Autodesk Fusion 360 part; units mm, degrees
sketch "Sketch1" plane through (0, 0, 0) normal (1, 0, 0) x (0, 1, 0)
  line L0 (28, -18) -> (-28, -18)
  line L1 (-28, 18) -> (28, 18)
  line L2 (28, -18) -> (-28, 18) construction
  line L3 (-28, -18) -> (28, 18) construction
  circle A0 centre (-28, 0) radius 8
  circle A1 centre (28, 0) radius 8
  arc A2 (-28, 18) -> (-28, -18) centre (-28, 0) ccw
  arc A3 (28, -18) -> (28, 18) centre (28, 0) ccw
  dimension "d1" = 56
  dimension "d2" = 36
  dimension "d3" = 36
  dimension "d4" = 36
  dimension "d5" = 16
  dimension "d6" = 16
extrude "Extrude1" add sketch "Sketch1" along normal blind 8
sketch "Sketch2" plane through (8, 0, 0) normal (1, 0, 0) x (0, 1, 0)
  circle A0 centre (-28, 0) radius 8
  circle A1 centre (28, 0) radius 8
  arc A2 (-28, 18) -> (-28, -18) centre (-28, 0) ccw
  line L0 (-28, -18) -> (28, -18)
  arc A3 (28, -18) -> (28, 18) centre (28, 0) ccw
  line L1 (28, 18) -> (-28, 18)
  line L2 (20, 8) -> (-20, 8)
  line L3 (-20, 8) -> (-20, 18)
  line L4 (20, 18) -> (20, 8)
extrude "Extrude2" add sketch "Sketch2" along normal blind 32 contours L1 L2 L3 L4
sketch "Sketch3" plane through (40, 0, 0) normal (1, 0, 0) x (0, 1, 0)
  line L0 (20, 18) -> (-20, 18)
  line L1 (-20, 18) -> (-20, 8)
  line L2 (-20, 8) -> (20, 8)
  line L3 (20, 8) -> (20, 18)
  circle A0 centre (0, 50) radius 10
  line L4 (-20, 18) -> (-14.832, 52.2387)
  line L5 (20, 18) -> (14.832, 52.2387)
  arc A1 (14.832, 52.2387) -> (-14.832, 52.2387) centre (0, 50) ccw
  dimension "d12" = 30
  dimension "d13" = 20
  dimension "d14" = 32
extrude "Extrude3" add sketch "Sketch3" against normal blind 10 contours L0 L4 L5 A1
sketch "Sketch4" plane through (40, 0, 0) normal (1, 0, 0) x (0, 1, 0)
  circle A0 centre (0, 50) radius 10
  line L0 (-20, 18) -> (-20, 8)
  line L1 (-20, 8) -> (20, 8)
  line L2 (20, 8) -> (20, 18)
  line L3 (20, 18) -> (14.832, 52.2387)
  arc A1 (14.832, 52.2387) -> (-14.832, 52.2387) centre (0, 50) ccw
  line L4 (-14.832, 52.2387) -> (-20, 18)
  circle A2 centre (0, 50) radius 15
  dimension "d17" = 30
extrude "Extrude4" add sketch "Sketch4" along normal blind 10 contours A1 A2
ref_plane "WorkPlane1" through (24, 0, 13) normal (0, -1, 0) x (0, 0, -1)
sketch "Sketch5" plane through (0, 0, 0) normal (0, -1, 0) x (-1, 0, 0)
  line L0 (-40, -8) -> (-8, 18)
  line L1 (-8, 18) -> (-8, -8)
  line L2 (-8, -8) -> (-40, -8)
  point P0 (-40, -8)
  point P1 (-8, -8)
  point P2 (-8, 18)
extrude "Extrude5" add sketch "Sketch5" along normal blind 6 and the other way blind 6
Can you work these out from the model? Positions are in its coordinate system, mm. A direction names the side the tool comes from. Coordinates: 2 decimals unless noted, no trailing zeros. Write each loop counter-clockwise with the first axis right and the second up, starting at its lowest first coordinate (ties: lowest second). Pieces come first, ordered by that corner, then holes. Notation, with made-up numbers: (9.5, 30.25) - (20.5, 30.25) arc R23 cw to (20.5, 67.25) - close; hole circle Ø5 at (46, 74.25). An arc over 180 degrees is marked (long way). Return JSON: item names as keys, results as strings. Group by question number.
Item 1: If we section it at B-B (x = 5.5): Write out the boundary of the cut face in (y, z), then the cut area to 3 significant figures.
Item 2: If we section it at A-A (y = 0): Write out the boundary of the cut face in (x, z), then the cut area to 3 significant figures.
Item 3: I'm going to push flat-ended pins straight in: pin 1 Ø21 at (x, z) = (30, -5.5) entering from +Y; pin 2 Ø2 at (y, z) = (3.5, 39) entering from -X; pin 3 Ø5 at (x, z) = (20.5, 13.5) entering from -Y; pin 4 Ø12 at (y, z) = (0, 50) entering from +X. Where does each tip first touch, or does it pass through?
Item 4: If we section it at C-C (z = 0): Write out the boundary of the cut face in (x, y).
Item 5: Please list where these lines run through material, in increasing order: probe 1 along Z at (x, y) = (41, 0); probe 2 along X at (y, z) = (18, 9); probe 3 along Z at (x, y) = (4, -28).
Item 6: If we section it at D-D (z = 48.5): Write out the boundary of the cut face in (x, y), then the cut area to 3 significant figures.
Item 7: We'd pull the mould along Y, two halves only. Please class faces 1 (the face through (24, 13, 8)), 2 (the face through (4, -36, 0)), 3 (the face through (17, 6, 1)): pulls with the +Y half, pulls with the -Y half, needs draft (parallel to the pull), parting line crosses it, or undercut.
Item 8: Which directions (+Z, -Z, +X, -X, +Y, -Y) give clear straight access to the entire face, cutting with the end or side of a thin tool? Please do faces 4 (the face through (30, 0, 37)), 5 (the face through (24, -13, 8)), 6 (the face through (24, -20, 13)), 7 (the face through (42.082, -3.252, 64.643)).
Return value:
{
 "1": {"outline": "(-28, -18) - (28, -18) arc R18 ccw to (28, 18) - (-28, 18) arc R18 ccw to start; hole circle Ø16 at (-28, 0); hole circle Ø16 at (28, 0)", "area": "2,630 mm^2"},
 "2": {"outline": "(0, -18) - (8, -18) - (40, 8) - (40, 35) - (50, 35) - (50, 40) - (30, 40) - (30, 18) - (0, 18) - close; (30, 60) - (50, 60) - (50, 65) - (30, 65) - close", "area": "1,390 mm^2"},
 "3": {"pin 1": "stops at y = 6", "pin 2": "stops at x = 30", "pin 3": "stops at y = -20", "pin 4": "passes through"},
 "4": {"outline": "(0, -46) - (8, -46) - (8, -36) - (0, -36) - close; (0, -20) - (8, -20) - (8, -6) - (30.15, -6) - (30.15, 6) - (8, 6) - (8, 20) - (0, 20) - close; (0, 36) - (8, 36) - (8, 46) - (0, 46) - close"},
 "5": {"probe 1": "z = 35 to 40, 60 to 65", "probe 2": "x = 0 to 40", "probe 3": "z = -18 to -8, 8 to 18"},
 "6": {"outline": "(30, -15.4) - (40, -15.4) - (40, -14.92) - (50, -14.92) - (50, -9.89) - (30, -9.89) - close; (30, 9.89) - (50, 9.89) - (50, 14.92) - (40, 14.92) - (40, 15.4) - (30, 15.4) - close", "area": "211 mm^2"},
 "7": {"face 1": "needs draft", "face 2": "undercut", "face 3": "pulls with the +Y half"},
 "8": {"face 4": "+Z, -X, +Y, -Y", "face 5": "-Z, +X, -Y", "face 6": "+Z, -Z, +X, -Y", "face 7": "+X"}
}
